Read the model definition and answer for the solid it produces. Units are mm, in the model's axes. A direction names the side the tool comes from. Give positions to 0.01 mm unless a question says otherwise; leave off trailing zeros. Loops run counter-clockwise (first coordinate to the right, second up) from the corner with the lowest first, then second, coordinate; pieces in that order, holes last. Notation, with made-up numbers: (52.25, 12.25) - (91.25, 12.25) arc R24 cw to (91.25, 41.25) - close; hole circle Ø4 at (3.25, 51.5). An arc over 180 degrees is marked (long way). Write item = value, one per line. Start each with the question number.
from build123d import *

# Parameters (mm, degrees)
F3_DEPTH      = 2.38125
F3_DEPTH_BACK = 2.38125
F5_DEPTH      = 12.7


with BuildPart() as f1:
    # F0 (on Front) → F1 (revolve)
    with BuildSketch(Plane.XZ):
        Polygon((12.7, 6.35), (0, 6.35), (0, 0), (152.4, 0), (152.4, 12.7), (146.05, 12.7), (146.05, 7.9375), (28.575, 7.9375), (28.575, 6.3373), (26.9748, 6.3373), (26.9748, 7.9375), (12.7, 7.9375), align=None)
    revolve(axis=Axis((76.2, 0, 0), (1, 0, 0)))

    # F2 (on Front) → F3 (cut, two sides)
    with BuildSketch(Plane.XZ) as f3_sk:
        with BuildLine():
            Line((104.5209977589, 15.0908644997), (69.8499977589, 15.0908644997))
            Line((69.8499977589, 15.0908644997), (69.8499977589, 8.7408644997))
            ThreePointArc((69.8499977589, 8.7408644997), (70.7799337286, 6.4958004694), (73.0249977589, 5.5658644997))
            Line((73.0249977589, 5.5658644997), (101.3459977589, 5.5658644997))
            ThreePointArc((101.3459977589, 5.5658644997), (103.5910617891, 6.4958004694), (104.5209977589, 8.7408644997))
            Line((104.5209977589, 8.7408644997), (104.5209977589, 15.0908644997))
        make_face()
    extrude(amount=-F3_DEPTH, mode=Mode.SUBTRACT)
    extrude(f3_sk.sketch, amount=F3_DEPTH_BACK, mode=Mode.SUBTRACT)

    # F4 (on face) → F5 (cut, through all)
    with BuildSketch(Plane(origin=(0, 0, 0), x_dir=(0, -1, 0), z_dir=(-1, 0, 0))):
        with BuildLine():
            Line((-6.35, 0), (-3.175, 5.499261314))
            ThreePointArc((-3.175, 5.499261314), (-5.499261314, 3.175), (-6.35, 0))
        make_face()
        with BuildLine():
            ThreePointArc((3.175, 5.499261314), (0, 6.35), (-3.175, 5.499261314))
            Line((-3.175, 5.499261314), (3.175, 5.499261314))
        make_face()
        with BuildLine():
            ThreePointArc((6.35, 0), (5.499261314, 3.175), (3.175, 5.499261314))
            Line((3.175, 5.499261314), (6.35, 0))
        make_face()
        with BuildLine():
            ThreePointArc((3.175, -5.499261314), (5.499261314, -3.175), (6.35, 0))
            Line((6.35, 0), (3.175, -5.499261314))
        make_face()
        with BuildLine():
            Line((3.175, -5.499261314), (-3.175, -5.499261314))
            ThreePointArc((-3.175, -5.499261314), (0, -6.35), (3.175, -5.499261314))
        make_face()
        with BuildLine():
            Line((-3.175, -5.499261314), (-6.35, 0))
            ThreePointArc((-6.35, 0), (-5.499261314, -3.175), (-3.175, -5.499261314))
        make_face()
    extrude(amount=-F5_DEPTH, mode=Mode.SUBTRACT)


solid = f1.part
1. For a pull along X with two mould halves and no side action, classify faces 1 (the flat face through (152.4, 0, 0)), 2 (the cylindrical face through (27.764, 3.856, -5.029)), 3 (the flat face through (0, 0, 0)) as released by +X, released by -X, zero draft, split by the parting line, or undercut.
2. A cutting plane is placed at C-C on x = 57. Give the vertices of the cut face in (y, z) (1 decimal).
3. Given P1, Ø4, axis at x = 88, y = 1, coming from the +Z side; P2, Ø1, axis at x = 93, z = 6.5, coming from the +Y side; P3, Ø1.5, axis at x = 78.5, y = -6.5, coming from the -Z side; P4, Ø8, axis at y = -1, z = 2.5, coming from the -X side, each flat-ended and moving along its own axis, determine where each tip first touches the part or whether it passes through.
4. A tool of negligible diameter and unlimited length cuts with its end or side. For faces 4 (the flat face through (6, 0, 5.499)), 5 (the flat face through (28.575, 6, -3)), 6 (the flat face through (6.26, -4.74, 2.79)), 7 (the cylindrical face through (103.26, 0.03, 6.21)), from which of +Z, -Z, +X, -X, +Y, -Y can it reach the whole face along a straight path? Write none if from no direction.
5. Consider line 1 along Y through (x, z) = (99, 0.25); line 2 along Z through (x, y) = (81, 4.75); line 3 along X through (y, z) = (11, 2.75). Determine where each line is inside the solid, lowest interval first. Write a range as [from, to].
6. A cutting plane is placed at D-D on z = 2.75. Give the vertices of the cut face in (x, y) (3 decimals), and give its area (3 significant figures).
7. A cutting plane is placed at B-B on z = -3. Give the vertices of the cut face in (x, y) (3 decimals).
Reply:
q1.face_1 = released by +X
q1.face_2 = undercut
q1.face_3 = released by -X
q2.outline = circle Ø15.9 at (0, 0)
q3.P1 = 7.57
q3.P2 = 5.2
q3.P3 = -5.47
q3.P4 = 0
q4.face_4 = +Z, -X, +Y, -Y
q4.face_5 = none
q4.face_6 = +Z, -X, -Y
q4.face_7 = +Z
q5.line_1 = [-7.93, 7.93]
q5.line_2 = [-6.36, 6.36]
q5.line_3 = [146.05, 152.4]
q6.outline = (0, -4.762) - (12.7, -4.762) - (12.7, -7.446) - (26.975, -7.446) - (26.975, -5.71) - (28.575, -5.71) - (28.575, -7.446) - (146.05, -7.446) - (146.05, -12.399) - (152.4, -12.399) - (152.4, 12.399) - (146.05, 12.399) - (146.05, 7.446) - (28.575, 7.446) - (28.575, 5.71) - (26.975, 5.71) - (26.975, 7.446) - (12.7, 7.446) - (12.7, 4.762) - (0, 4.762) - close
q6.area = 2,260 mm^2
q7.outline = (0, -4.618) - (12.7, -4.618) - (12.7, -7.349) - (26.975, -7.349) - (26.975, -5.582) - (28.575, -5.582) - (28.575, -7.349) - (146.05, -7.349) - (146.05, -12.341) - (152.4, -12.341) - (152.4, 12.341) - (146.05, 12.341) - (146.05, 7.349) - (28.575, 7.349) - (28.575, 5.582) - (26.975, 5.582) - (26.975, 7.349) - (12.7, 7.349) - (12.7, 4.618) - (0, 4.618) - close
